Geometry check sheet. Reference: the model listing, model coordinates, mm. Round coordinates to 2 decimals unless told otherwise and drop trailing zeros. Order: outer loops, then holes, each group sorted by start corner. A loop starts at its lowest first (then second) coordinate and runs counter-clockwise, first axis right, second up. Notation, with made-up numbers: (36.5, 24) - (78.5, 24) arc R20 cw to (78.5, 37) - close; hole circle Ø3 at (53, -2.75). An arc over 180 degrees is marked (long way). Return JSON: item names as keys, results as strings. Group by question number.
Q1. Sectioned sample at B-B, the plane z = 16.8. Record the cut outline in (x, y).
Q2. Gauge pin test, flat ends, axial feed: pin 1 Ø0.9 at (y, z) = (1, -19) entering from +X; pin 2 Ø0.9 at (x, y) = (19, 1.5) entering from -Z; pin 3 Ø1 at (x, z) = (-9.5, -15.5) entering from -Y. Record the tip position at first contact, or that the pin passes through.
Q3. Sectioned sample at C-C, the plane x = -1. Record the cut outline in (y, z), then the cut area to 3 significant figures.
Q4. Material ranges on line 1 along X through (y, z) = (1.2, 16.8); line 2 along Z through (x, y) = (-3.5, 0.55); line 3 along Z through (x, y) = (-5, 0.75), recorded low to high.
Q5. Sectioned sample at A-A, the plane x = -7.6. Record the cut outline in (y, z).
Q6. Sectioned sample at D-D, the plane y = 0.7. Record the cut outline in (x, z), then the cut area to 3 significant figures.
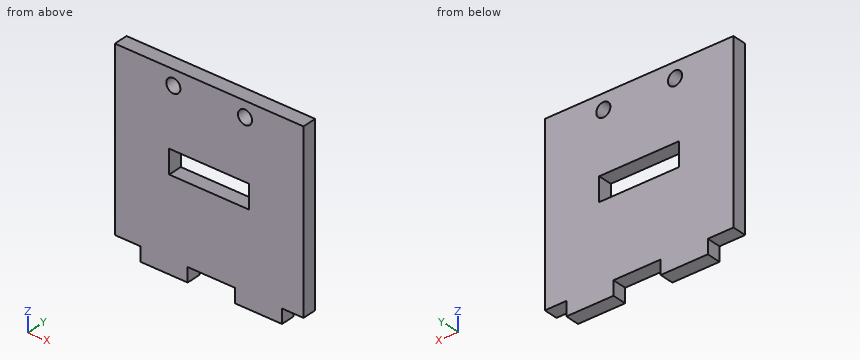
```python
from build123d import *

# Parameters (mm, degrees)
SKETCH1_W           = 40
SKETCH1_H           = 40
BOSS_EXTRUDE1_DEPTH = 3
SKETCH2_R           = 1.5
SKETCH2_W           = 16.950963154
SKETCH2_H           = 5
CUT_EXTRUDE2_DEPTH  = 10
CUT_EXTRUDE3_DEPTH  = 10


with BuildPart() as part:
    # Sketch1 → Boss-Extrude1 (new body)
    with BuildSketch(Plane(origin=(0, 0, 0), x_dir=(1, 0, 0), z_dir=(0, 1, 0))):
        Rectangle(SKETCH1_W, SKETCH1_H)
    extrude(amount=BOSS_EXTRUDE1_DEPTH)

    # Sketch2 → Cut-Extrude2 (cut)
    with BuildSketch(Plane.XZ):
        with Locations(Location((7.6, 16.8, 0), (0, 0, 270))):
            Circle(SKETCH2_R)
        with Locations(Location((-7.6, 16.8, 0), (0, 0, 270))):
            Circle(SKETCH2_R)
        with Locations((0, 1.8)):
            Rectangle(SKETCH2_W, SKETCH2_H)
    extrude(amount=-CUT_EXTRUDE2_DEPTH, mode=Mode.SUBTRACT)

    # Sketch5 → Cut-Extrude3 (cut)
    with BuildSketch(Plane.XZ):
        Polygon((20, -17), (15.444490667, -17), (15.444490667, -20), (5.444490667, -20), (5.444490667, -17), (-4.555509333, -17), (-4.555509333, -20), (-14.555509333, -20), (-14.555509333, -17), (-20, -17), (-20, -21.558033771), (20, -21.558033771), align=None)
    extrude(amount=-CUT_EXTRUDE3_DEPTH, mode=Mode.SUBTRACT)


solid = part.part
```
Reply:
{
 "1": {"outline": "(-20, 0) - (-9.1, 0) - (-9.1, 3) - (-20, 3) - close; (-6.1, 0) - (6.1, 0) - (6.1, 3) - (-6.1, 3) - close; (9.1, 0) - (20, 0) - (20, 3) - (9.1, 3) - close"},
 "2": {"pin 1": "x = 15.44", "pin 2": "z = -17", "pin 3": "y = 0"},
 "3": {"outline": "(0, -17) - (3, -17) - (3, -0.7) - (0, -0.7) - close; (0, 4.3) - (3, 4.3) - (3, 20) - (0, 20) - close", "area": "96.0 mm^2"},
 "4": {"line 1": "-20 to -9.1, -6.1 to 6.1, 9.1 to 20", "line 2": "-17 to -0.7, 4.3 to 20", "line 3": "-20 to -0.7, 4.3 to 20"},
 "5": {"outline": "(0, -20) - (3, -20) - (3, -0.7) - (0, -0.7) - close; (0, 4.3) - (3, 4.3) - (3, 15.3) - (0, 15.3) - close; (0, 18.3) - (3, 18.3) - (3, 20) - (0, 20) - close"},
 "6": {"outline": "(-20, -17) - (-14.56, -17) - (-14.56, -20) - (-4.56, -20) - (-4.56, -17) - (5.44, -17) - (5.44, -20) - (15.44, -20) - (15.44, -17) - (20, -17) - (20, 20) - (-20, 20) - close; hole circle Ø3 at (-7.6, 16.8); hole (-8.48, -0.7) - (8.48, -0.7) - (8.48, 4.3) - (-8.48, 4.3) - close; hole circle Ø3 at (7.6, 16.8)", "area": "1,440 mm^2"}
}
